Input: part model. Units: mm. Frame: model coordinates. A direction names the side the tool comes from. Give positions to 0.01 mm unless a question says otherwise; leave off trailing zeros. Write each loop counter-clockwise with the first axis right and the second up, starting at its lowest first coordinate (ties: lowest second). Pieces come first, ordered by that corner, then holes. Notation, with made-up numbers: (46.5, 72.25) -> (79.5, 72.25) arc R23 cw to (79.5, 108.25) -> close; hole circle Ø10 at (40.25, 21). An arc over 180 degrees is marked (long way). Return JSON: item names as keys, results as strings. Group by question number.
Item 1: Pin query (flat end, axial travel): P1, Ø2.5, axis at x = 48.5, y = 6, coming from the +Z side; P2, Ø1, axis at x = 29, y = 2, coming from the +Z side; P3, Ø3.5, axis at x = 47, z = 4.5, coming from the +Y side. Return the tip coordinate at first contact, or that it passes through.
Item 2: Section B-B, the plane x = 33. Return loops of the section in (y, z).
Item 3: Mould query, pull axis Y, two halves, no side actions, for faces 4 (the face through (-1, -1.661, 4)), 5 (the face through (-1, -0.261, 5)), 6 (the face through (1.4, 4.6, 2)). Classes: released by +Y, released by -Y, zero draft, split by the parting line, or undercut.
Item 4: Section A-A, the plane z = 6. Return loops of the section in (x, y).
Item 5: Set-up query: faces 1 (the face through (-100, 3, 2)), 2 (the face through (-1, 1.939, 5)), 3 (the face through (-1, 3.339, 5)). Return all of +Z, -Z, +X, -X, +Y, -Y with unobstructed straight access to the full face (end or side cutting, diameter ignored); none if empty.
Item 6: Line query: line 1 (Y direction, x = -48, z = 5.5); line 2 (Y direction, x = 0, z = 0.2); line 3 (X direction, y = 7, z = 0.75). Output: solid intervals per line, ascending. Write a range as [from, to].
from build123d import *

# Parameters (mm, degrees)
F0_W           = 200
F0_H           = 5
F1_DEPTH       = 8.5
F2_W           = 200
F2_H           = 2.2
F3_DEPTH       = 5.5
F4_W           = 200
F4_H           = 2
F5_DEPTH       = 8
F7_D           = 2.5
F7_CSINK_D     = 5
F7_CSINK_ANGLE = 90
F8_SIZE        = 1


with BuildPart() as f1:
    # F0 (on Top) → F1 (new body)
    with BuildSketch(Plane.XY):
        with Locations((0, 0.839391)):
            Rectangle(F0_W, F0_H)
    extrude(amount=F1_DEPTH)

    # F2 (on face) → F3 (cut)
    with BuildSketch(Plane.XY.offset(8.5)):
        with Locations((0, 0.839391)):
            Rectangle(F2_W, F2_H)
    extrude(amount=-F3_DEPTH, mode=Mode.SUBTRACT)

    # F4 (on face) → F5 (join)
    with BuildSketch(Plane(origin=(0, 3.339391, 0), x_dir=(-1, 0, 0), z_dir=(0, 1, 0))):
        with Locations((0, 1)):
            Rectangle(F4_W, F4_H)
    extrude(amount=F5_DEPTH)

    # F7 (through all)
    with Locations(Plane.XY.offset(2)):
        with Locations((0, 7.339391), (80, 7.339391), (-80, 7.339391)):
            CounterSinkHole(F7_D / 2, F7_CSINK_D / 2, counter_sink_angle=F7_CSINK_ANGLE)

    # F8
    f8_edges = [f1.edges().sort_by_distance(p)[0] for p in [
        (0, 1.939391, 8.5),
        (0, -0.260609, 8.5),
    ]]
    chamfer(f8_edges, length=F8_SIZE)


solid = f1.part
Answer below:
{
 "1": {"P1": "stops at z = 2", "P2": "stops at z = 8.06", "P3": "stops at y = 3.34"},
 "2": {"outline": "(-1.66, 0) -> (11.34, 0) -> (11.34, 2) -> (3.34, 2) -> (3.34, 8.5) -> (2.94, 8.5) -> (1.94, 7.5) -> (1.94, 3) -> (-0.26, 3) -> (-0.26, 7.5) -> (-1.26, 8.5) -> (-1.66, 8.5) -> close"},
 "3": {"face 4": "released by -Y", "face 5": "undercut", "face 6": "zero draft"},
 "4": {"outline": "(-100, -1.66) -> (100, -1.66) -> (100, -0.26) -> (-100, -0.26) -> close; (-100, 1.94) -> (100, 1.94) -> (100, 3.34) -> (-100, 3.34) -> close"},
 "5": {"face 1": "+Z, -Z, -X, +Y, -Y", "face 2": "+Z, +X, -X", "face 3": "+Z, +X, -X, +Y"},
 "6": {"line 1": "y = [-1.66, -0.26], [1.94, 3.34]", "line 2": "y = [-1.66, 6.09], [8.59, 11.34]", "line 3": "x = [-100, -81.2], [-78.8, -1.2], [1.2, 78.8], [81.2, 100]"}
}
